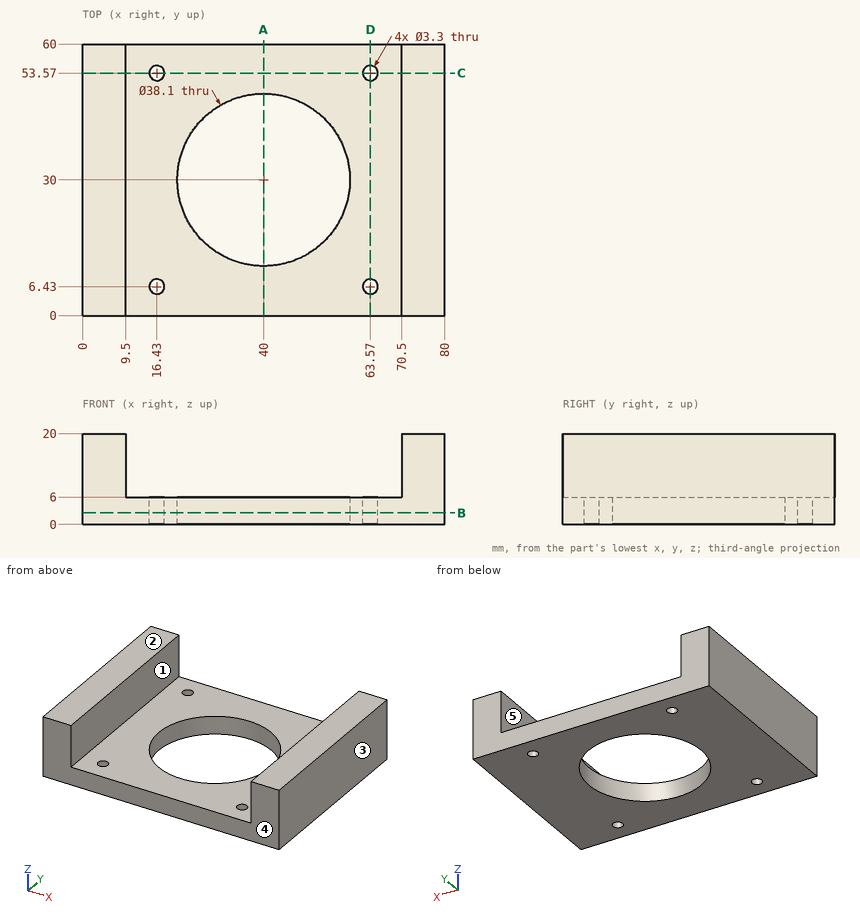
Verification items for this drawing (mm, ordinates from the low corner). A direction names the side the tool comes from. Give positions to 0.01 mm unless a question says otherwise; leave off trailing zeros. Order: outer loops, then holes, each group sorted by start corner. A loop starts at its lowest first (then second) coordinate and runs counter-clockwise, first axis right, second up.
1) Material ranges on probe 1 along Y at (x, z) = (63.57, 4.65); probe 2 along X at (y, z) = (34, 16.5); probe 3 along Y at (x, z) = (40, 2), recorded low to high.
Results are:
probe 1: y = 0 to 4.78, 8.08 to 51.92, 55.22 to 60
probe 2: x = 0 to 9.5, 70.5 to 80
probe 3: y = 0 to 10.95, 49.05 to 60
2) Gauge pin test, flat ends, axial feed: pin 1 (10 mm diameter, centred on x = 57, y = 21, fed in from +Z); pin 2 (12 mm diameter, centred on x = 41, z = 8.5, fed in from +Y); pin 3 (2.5 mm diameter, centred on x = 16.43, y = 6.43, fed in from +Z). Record the tip position at first contact, or that the pin passes through.
Results are:
pin 1: stops at z = 6
pin 2: stops at y = 60
pin 3: passes through
3) Cross-section at B-B (z = 2.5). Record the boundary of the cut face in (x, y).
Results are:
outline: (0, 0) - (80, 0) - (80, 60) - (0, 60) - close; hole circle Ø3.3 at (16.43, 6.43); hole circle Ø3.3 at (16.43, 53.57); hole circle Ø38.1 at (40, 30); hole circle Ø3.3 at (63.57, 6.43); hole circle Ø3.3 at (63.57, 53.57)
4) Tool access check on the marked faces 4 and 5. Record the directions out of +Z, -Z, +X, -X, +Y, -Y that give a thin tool (end or side, any length) a straight path to the whole face; none if there is none.
Results are:
face 4: +Z, -Z, +X, -X, -Y
face 5: +Z, +Y, -Y
5) Cross-section at D-D (x = 63.57). Record the boundary of the cut face in (y, z).
Results are:
outline: (0, 0) - (4.78, 0) - (4.78, 6) - (0, 6) - close; (8.08, 0) - (51.92, 0) - (51.92, 6) - (8.08, 6) - close; (55.22, 0) - (60, 0) - (60, 6) - (55.22, 6) - close
6) Cross-section at C-C (y = 53.57). Record the boundary of the cut face in (x, z), then the cut area to 3 significant figures.
Results are:
outline: (0, 0) - (14.78, 0) - (14.78, 6) - (9.5, 6) - (9.5, 20) - (0, 20) - close; (18.08, 0) - (61.92, 0) - (61.92, 6) - (18.08, 6) - close; (65.22, 0) - (80, 0) - (80, 20) - (70.5, 20) - (70.5, 6) - (65.22, 6) - close
area: 706 mm2
7) Draft check along X on the marked faces 1, 2 and 3. Enter one of: released by +X, released by -X, zero draft, split by the parting line, or undercut.
Results are:
face 1: undercut
face 2: zero draft
face 3: released by +X
8) Cross-section at A-A (x = 40). Record the boundary of the cut face in (y, z).
Results are:
outline: (0, 0) - (10.95, 0) - (10.95, 6) - (0, 6) - close; (49.05, 0) - (60, 0) - (60, 6) - (49.05, 6) - close
